Build history of the part. All positions in model axes, mm. Round coordinates to 2 decimals unless told otherwise and drop trailing zeros. Write each loop counter-clockwise with the first axis right and the second up, starting at its lowest first coordinate (ties: lowest second). Pieces come first, ordered by that corner, then holes. Notation, with made-up numbers: (86, 68.25) -> (108, 68.25) arc R19 ccw to (108, 77.25) -> close; hole circle Ø10 at (80.5, 28). An arc over 180 degrees is marked (long way). One line per question, with ' | ' between items.
from build123d import *

# Parameters (mm, degrees)
SKETCH1_W           = 14
SKETCH1_H           = 241
BOSS_EXTRUDE1_DEPTH = 5
CUT_EXTRUDE3_REACH  = 243.458
SKETCH4_W           = 2
SKETCH4_H           = 217
CUT_EXTRUDE1_DEPTH  = 242.458070894
CUT_EXTRUDE2_DEPTH  = 2
FILLET1_R           = 1


with BuildPart() as part:
    # Sketch1 → Boss-Extrude1 (new body)
    with BuildSketch(Plane.XY):
        with Locations((7, 120.5)):
            Rectangle(SKETCH1_W, SKETCH1_H)
    extrude(amount=BOSS_EXTRUDE1_DEPTH)

    # Sketch4 → Cut-Extrude3 (cut, up to next)
    with BuildSketch(Plane.XY.offset(5), mode=Mode.PRIVATE) as cut_extrude3_sk1:
        with Locations((1, 120.5)):
            Rectangle(SKETCH4_W, SKETCH4_H)
    cut_extrude3_tool1 = extrude(cut_extrude3_sk1.sketch, amount=-CUT_EXTRUDE3_REACH, mode=Mode.PRIVATE) & part.part
    # Sketch4 → Cut-Extrude3 (cut, up to next)
    with BuildSketch(Plane.XY.offset(5), mode=Mode.PRIVATE) as cut_extrude3_sk2:
        with Locations((13, 120.5)):
            Rectangle(SKETCH4_W, SKETCH4_H)
    cut_extrude3_tool2 = extrude(cut_extrude3_sk2.sketch, amount=-CUT_EXTRUDE3_REACH, mode=Mode.PRIVATE) & part.part
    add(cut_extrude3_tool1.solids().sort_by_distance((1, 120.5, 5))[0], mode=Mode.SUBTRACT)
    add(cut_extrude3_tool2.solids().sort_by_distance((13, 120.5, 5))[0], mode=Mode.SUBTRACT)

    # Sketch2 → Cut-Extrude1 (cut, through all)
    with BuildSketch(Plane.XY.offset(5)):
        with BuildLine():
            Line((8.75, 7), (8.75, 5))
            ThreePointArc((8.75, 5), (7, 3.25), (5.25, 5))
            Line((5.25, 5), (5.25, 7))
            ThreePointArc((5.25, 7), (7, 8.75), (8.75, 7))
        make_face()
        with BuildLine():
            Line((8.75, 236), (8.75, 234))
            ThreePointArc((8.75, 234), (7, 232.25), (5.25, 234))
            Line((5.25, 234), (5.25, 236))
            ThreePointArc((5.25, 236), (7, 237.75), (8.75, 236))
        make_face()
    extrude(amount=-CUT_EXTRUDE1_DEPTH, mode=Mode.SUBTRACT)

    # Sketch3 → Cut-Extrude2 (cut)
    with BuildSketch(Plane.XY.offset(5)):
        with BuildLine():
            Line((9.75, 7), (9.75, 5))
            ThreePointArc((9.75, 5), (7, 2.25), (4.25, 5))
            Line((4.25, 5), (4.25, 7))
            ThreePointArc((4.25, 7), (7, 9.75), (9.75, 7))
        make_face()
        with BuildLine():
            Line((9.75, 236), (9.75, 234))
            ThreePointArc((9.75, 234), (7, 231.25), (4.25, 234))
            Line((4.25, 234), (4.25, 236))
            ThreePointArc((4.25, 236), (7, 238.75), (9.75, 236))
        make_face()
    extrude(amount=-CUT_EXTRUDE2_DEPTH, mode=Mode.SUBTRACT)

    # Fillet1
    fillet1_edges = [part.edges().sort_by_distance(p)[0] for p in [
        (2, 229, 2.5),
        (12, 229, 2.5),
        (12, 12, 2.5),
        (2, 12, 2.5),
    ]]
    fillet(fillet1_edges, radius=FILLET1_R)
    fillet1_2_edges = [part.edges().sort_by_distance(p)[0] for p in [
        (0, 241, 2.5),
        (14, 241, 2.5),
        (7, 241, 5),
        (14, 6, 5),
        (14, 235, 5),
        (0, 6, 5),
        (0, 235, 5),
        (7, 0, 5),
        (0, 0, 2.5),
        (14, 0, 2.5),
        (0, 229, 2.5),
        (14, 229, 2.5),
        (12, 120.5, 5),
        (14, 12, 2.5),
        (2, 120.5, 5),
        (0, 12, 2.5),
        (1.707106781, 228.707106781, 5),
        (1.707106781, 12.292893219, 5),
        (12.292893219, 228.707106781, 5),
        (12.292893219, 12.292893219, 5),
    ]]
    fillet(fillet1_2_edges, radius=FILLET1_R - 0.0001)  # a hair under: the kernel refuses the full size


solid = part.part
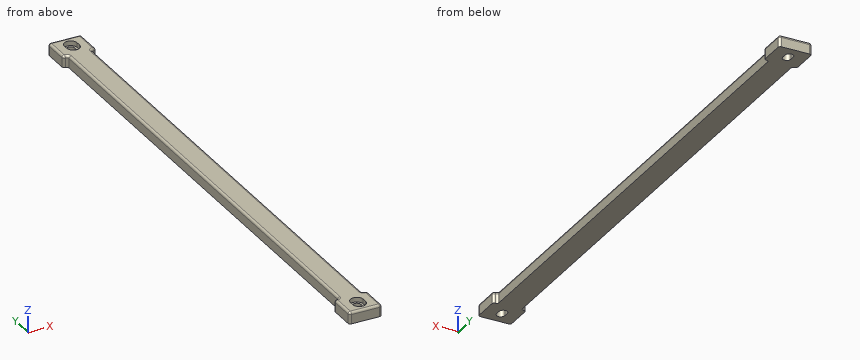
(1) Slice it at B-B (y = 21.5). Write the cut outline in (x, z).
Calculated:
outline: (2, 0) -> (12, 0) -> (12, 4) arc R1 ccw to (11, 5) -> (3, 5) arc R1 ccw to (2, 4) -> close
(2) Slice it at A-A (z = 0.8). State how many separate pieces and enclosed holes the cut face has, then the cut area to 3 significant figures.
Calculated:
separate pieces: 1 | enclosed holes: 2 | area: 2,470 mm2
(3) Drop flat-ended pins along their axis: pin 1 (1 mm diameter, centred on y = 182.5, z = 1, fed in from +X); pin 2 (1.6 mm diameter, centred on x = 6, y = 8, fed in from +Z); pin 3 (3 mm diameter, centred on y = 67, z = 1.5, fed in from -X); pin 4 (1.6 mm diameter, centred on x = 7, y = 234.5, fed in from +Z). Give the stop position or say it passes through.
Calculated:
pin 1: x = 12 | pin 2: z = 3 | pin 3: x = 2 | pin 4: through
(4) Wall check: line 1 (Y direction, x = 6.75, z = 1.75); line 2 (Y direction, x = 6.5, z = 3.15); line 3 (Y direction, x = 13.25, z = 2.45). Give the ranges that are in metal, low to high. Write a range as from..to.
Calculated:
line 1: 0..3.27, 8.73..232.27, 237.73..241 | line 2: 0..2.3, 9.7..231.3, 238.7..241 | line 3: 0.03..11.97, 229.03..240.97
